Can you work these out from the drawing? Everything is in mm from the part's minimum corner. A direction names the side the tool comes from. Give positions to 0.01 mm unless a question says otherwise; leave off trailing zeros. Write each loop counter-clockwise with the first axis right and the second up, starting at its lowest first coordinate (ties: lowest second). Pieces come first, ordered by that corner, then holes. Notation, with made-up numbers: (-35.5, -38.5) - (-24.5, -38.5) arc R14 cw to (-24.5, -18.5) - close; hole circle Ø2 at (-9, -3). An arc over 180 degrees is marked (long way). Return JSON: item names as keys, results as strings. Group by question number.
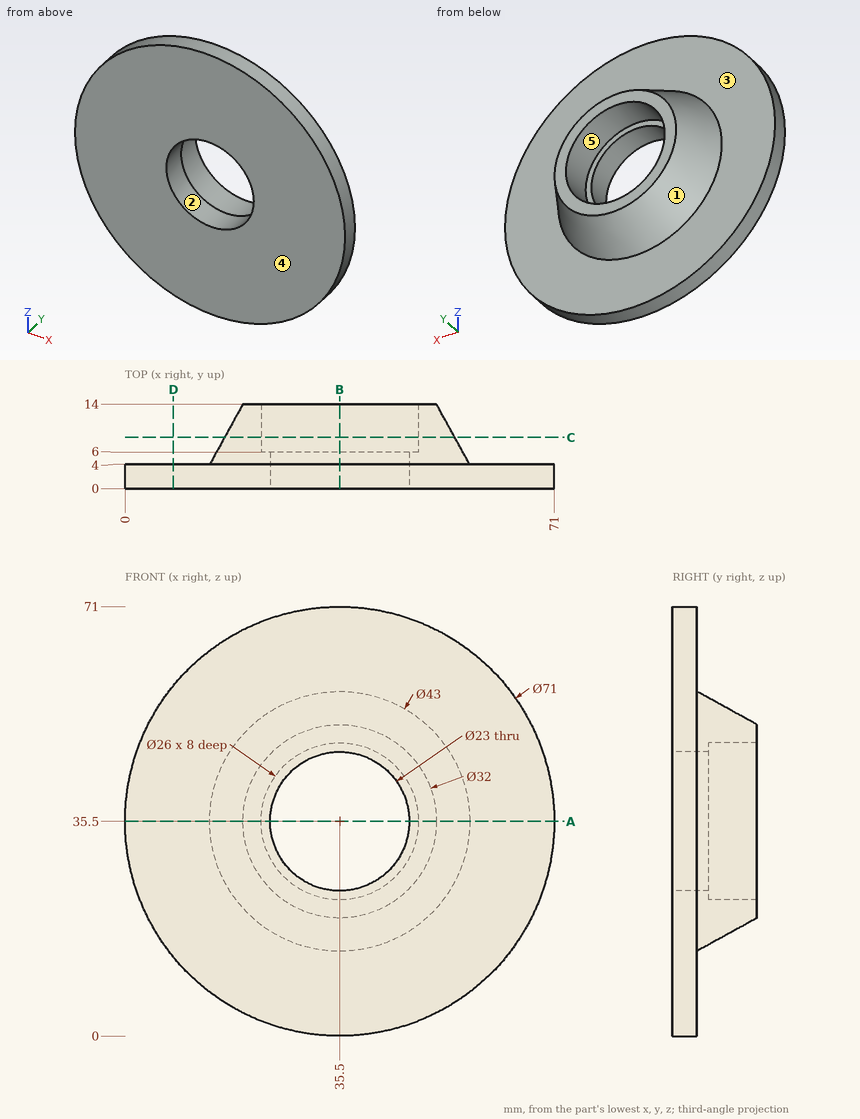
1) Imagine slicing it at A-A, the plane z = 35.5. Write out the boundary of the cut face in (x, y), and give its area (3 significant figures).
2) Imagine slicing it at D-D, the plane x = 8. Write out the boundary of the cut face in (y, z), and give its area (3 significant figures).
3) We'd pull the mould along Z, two halves only. Please class the marked faces 1, 2 and 3: pulls with the +Z half, pulls with the -Z half, needs draft (parallel to the pull), parting line crosses it, or undercut.
4) Will these pins go through, and if not, where does the flat tip stop? pin 1 Ø4 at (x, y) = (20, 4) entering from -Z; pin 2 Ø18.5 at (x, z) = (35.5, 35.5) entering from +Y; pin 3 Ø6 at (x, z) = (56, 58.5) entering from +Y; pin 4 Ø8 at (y, z) = (12, 30.5) entering from +X.
5) Imagine slicing it at C-C, the plane y = 8.5. Write out the boundary of the cut face in (x, z) (3 decimals), and give its area (3 significant figures).
6) On a 3-axis mill with a long thin cutter (end or side, diameter ignored), from which of +Z, -Z, +X, -X, +Y, -Y can I reach the whole of each face in a straight line? I mean the marked faces 4 and 5. Say none if no direction works.
7) Imagine slicing it at B-B, the plane x = 35.5. Write out the boundary of the cut face in (y, z).
8) I need wall thicknesses on line 1 along Z through (x, y) = (35.5, 3.7); line 2 along Y through (x, z) = (36.5, 14). Which ranges of each line are inside material? Lowest first, please.
Resolved:
{
 "1": {"outline": "(0, 0) - (24, 0) - (24, 6) - (22.5, 6) - (22.5, 14) - (19.5, 14) - (14, 4) - (0, 4) - close; (47, 0) - (71, 0) - (71, 4) - (57, 4) - (51.5, 14) - (48.5, 14) - (48.5, 6) - (47, 6) - close", "area": "313 mm^2"},
 "2": {"outline": "(0, 13.05) - (4, 13.05) - (4, 57.95) - (0, 57.95) - close", "area": "180 mm^2"},
 "3": {"face 1": "parting line crosses it", "face 2": "undercut", "face 3": "needs draft"},
 "4": {"pin 1": "z = 2.67", "pin 2": "through", "pin 3": "y = 4", "pin 4": "x = 54.32"},
 "5": {"outline": "circle Ø38.05 at (35.5, 35.5); hole circle Ø26 at (35.5, 35.5)", "area": "606 mm^2"},
 "6": {"face 4": "+Z, -Z, +X, -X, -Y", "face 5": "+Y"},
 "7": {"outline": "(0, 0) - (4, 0) - (4, 14) - (14, 19.5) - (14, 22.5) - (6, 22.5) - (6, 24) - (0, 24) - close; (0, 47) - (6, 47) - (6, 48.5) - (14, 48.5) - (14, 51.5) - (4, 57) - (4, 71) - (0, 71) - close"},
 "8": {"line 1": "0 to 24, 47 to 71", "line 2": "0 to 4"}
}
